Here's the drawing with two shaded views (mm, measured from the low corner). I have some questions. A direction names the side the tool comes from. Round coordinates to 2 decimals unless told otherwise and drop trailing zeros. Loops run counter-clockwise (first coordinate to the right, second up) from the corner with the lowest first, then second, coordinate; pieces in that order, holes last. Notation, with made-up numbers: M 72.5,74 L 90.5,74 A20 cw 90.5,108 Z; hole C 52.5,69.25 d7. An arc over 180 degrees is marked long. One line per item, written item: value. Start each with the question number.
Q1. I'm going to push flat-ended pins straight in: pin 1 Ø1.5 at (x, y) = (3, 4.5) entering from -Z; pin 2 Ø1 at (x, y) = (28, 7) entering from -Z; pin 3 Ø1.8 at (x, y) = (39, 15) entering from +Z. Where does each tip first touch, or does it pass through?
Q2. Which directions (+Z, -Z, +X, -X, +Y, -Y) give clear straight access to the entire face, cutting with the end or side of a thin tool? Please do the marked faces 1, 2 and 3.
Q3. Imagine slicing it at A-A (z = 12). Please give me the cut outline in (x, y), then the cut area to 3 significant figures.
Q4. Please list where these lines run through material, in increasing order: line 1 along X through (y, z) = (12, 10); line 2 along Y through (x, z) = (39, 4.5); line 3 along X through (y, z) = (15, 8).
Q5. Imagine slicing it at B-B (x = 39). Please give me the cut outline in (y, z), then the cut area to 3 significant figures.
Q6. Imagine slicing it at D-D (y = 10). Please give me the cut outline in (x, z), then the cut area to 3 significant figures.
Q7. Imagine slicing it at C-C (y = 7). Please give me the cut outline in (x, z), then the cut area to 3 significant figures.
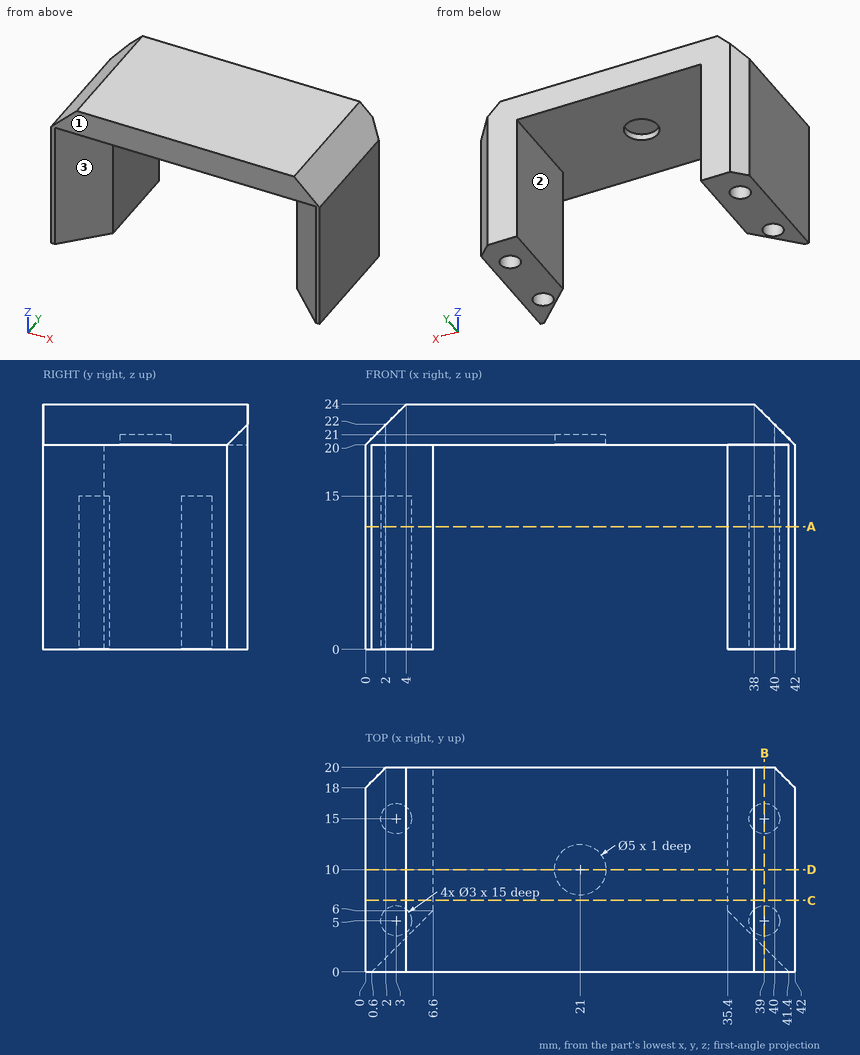
Report:
1. pin 1: stops at z = 15
1. pin 2: stops at z = 20
1. pin 3: stops at z = 23.9
2. face 1: +Z, -Z, +X, -X, -Y
2. face 2: -Z, +Y, -Y
2. face 3: -Z, -Y
3. outline: M 0,0 L 0.6,0 L 6.6,6 L 6.6,20 L 2,20 L 0,18 Z; M 35.4,6 L 41.4,0 L 42,0 L 42,18 L 40,20 L 35.4,20 Z; hole C 3,5 d3; hole C 3,15 d3; hole C 39,5 d3; hole C 39,15 d3
3. area: 196 mm²
4. line 1: x = 0 to 6.6, 35.4 to 42
4. line 2: y = 2.4 to 3.5, 6.5 to 13.5, 16.5 to 20
4. line 3: x = 0 to 1.5, 4.5 to 6.6, 35.4 to 37.5, 40.5 to 42
5. outline: M 0,20 L 2.4,20 L 2.4,0 L 3.5,0 L 3.5,15 L 6.5,15 L 6.5,0 L 13.5,0 L 13.5,15 L 16.5,15 L 16.5,0 L 20,0 L 20,23 L 0,23 Z
5. area: 322 mm²
6. outline: M 0,0 L 6.6,0 L 6.6,20 L 18.5,20 L 18.5,21 L 23.5,21 L 23.5,20 L 35.4,20 L 35.4,0 L 42,0 L 42,20 L 38,24 L 4,24 L 0,20 Z
6. area: 411 mm²
7. outline: M 0,0 L 6.6,0 L 6.6,20 L 35.4,20 L 35.4,0 L 42,0 L 42,20 L 38,24 L 4,24 L 0,20 Z
7. area: 416 mm²
